CAD build for the part. Positions are in the model's coordinates, mm. Round coordinates to 2 decimals unless told otherwise and drop trailing zeros. Loops run counter-clockwise (first coordinate to the right, second up) from the corner with the lowest first, then second, coordinate; pieces in that order, holes last. Notation, with made-up numbers: M 33.25,61 L 82.25,61 A31 ccw 82.25,95 Z; hole C 47.5,-36 d9. An arc over 180 degrees is marked long. Use one line per item in the form item = value.
from build123d import *

# Parameters (mm, degrees)
SKETCH_1_W          = 76.2
SKETCH_1_H          = 25.4
EXTRUDE_1_DEPTH     = 1
CUT_EXTRUDE_1_DEPTH = 1


with BuildPart() as part:
    # 草图1 → 凸台-拉伸1 (new body)
    with BuildSketch(Plane(origin=(0, 0, 0), x_dir=(1, 0, 0), z_dir=(0, 1, 0))):
        with Locations((38.1, -12.7)):
            Rectangle(SKETCH_1_W, SKETCH_1_H)
    extrude(amount=EXTRUDE_1_DEPTH)

    # 草图2 → 切除-拉伸1 (cut)
    with BuildSketch(Plane(origin=(0, 1, 0), x_dir=(1, 0, 0), z_dir=(0, 1, 0))):
        Polygon((3.55, -12.7), (3.55, -6.75), (15.45, -6.75), (15.45, -18.65), (3.55, -18.65), align=None)
    extrude(amount=-CUT_EXTRUDE_1_DEPTH, mode=Mode.SUBTRACT)


solid = part.part
1. Cut at C-C on y = 0.35. Write the cut outline in (x, z).
Completed:
outline = M 0,0 L 76.2,0 L 76.2,25.4 L 0,25.4 Z; hole M 3.55,6.75 L 15.45,6.75 L 15.45,18.65 L 3.55,18.65 Z
2. Cut at B-B on z = 10.5. Write the cut outline in (x, y), and give its area (3 significant figures).
Completed:
outline = M 0,0 L 3.55,0 L 3.55,1 L 0,1 Z; M 15.45,0 L 76.2,0 L 76.2,1 L 15.45,1 Z
area = 64.3 mm2
3. Cut at A-A on x = 13. Write the cut outline in (y, z), and give its area (3 significant figures).
Completed:
outline = M 0,0 L 1,0 L 1,6.75 L 0,6.75 Z; M 0,18.65 L 1,18.65 L 1,25.4 L 0,25.4 Z
area = 13.5 mm2
4. Probe line 1 along X through (y, z) = (0.7, 13). List the from-to ranges inside material, lowest first. Write a range as from..to.
Completed:
line_1 = 0..3.55, 15.45..76.2
